from build123d import *

# Parameters (mm, degrees)
SKETCH_2_R   = 4
SKETCH_2_R_2 = 3.5


with BuildPart() as part:
    # По траектории1: sweep along a path in Эскиз1
    with BuildLine(Plane.XY) as sweep_1_path:
        Line((-12.67059026, 57.046486939), (-18.171515217, 27.990319213))
        ThreePointArc((-18.171515217, 27.990319213), (-18.041069279, 23.679327915), (-16.107188295, 19.824231748))
        Line((-16.107188295, 19.824231748), (-6.305926251, 7.761140001))
        Line((-6.305926251, 7.761140001), (0, 0))
    # Эскиз2 → По траектории1 (sweep)
    with BuildSketch(Plane(origin=(0, 0, 0), x_dir=(-0.7761140001162656, -0.6305926250944656, 0), z_dir=(0.6305926250944656, -0.7761140001162656, 0))):
        Circle(SKETCH_2_R)
        Circle(SKETCH_2_R_2, mode=Mode.SUBTRACT)
    sweep(path=sweep_1_path.line)


solid = part.part
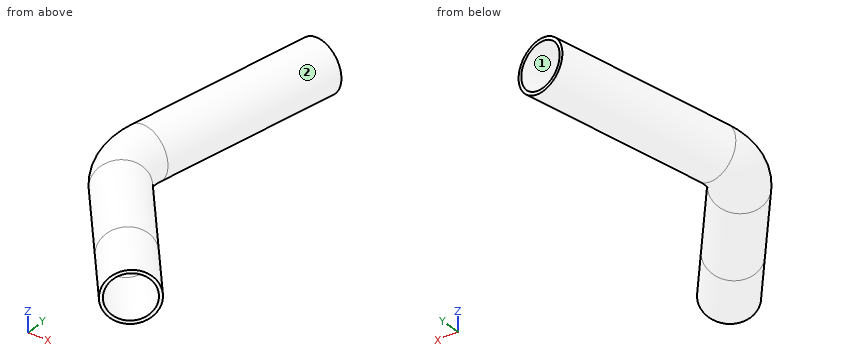
Input: part model. Units: mm. Frame: model coordinates. Face numbers are marked on the shaded views. Give positions to 0.01 mm unless a question says otherwise; leave off trailing zeros. Write each loop counter-clockwise with the first axis right and the second up, starting at its lowest first coordinate (ties: lowest second). Pieces come first, ordered by that corner, then holes. Notation, with made-up numbers: (-31, 3) -> (-26, 3) arc R23 cw to (-26, 22) -> close; hole circle Ø5 at (33.25, 69.25). An arc over 180 degrees is marked (long way). Use one line per item in the form item = value. Start each with the question number.
1) Ray query, probe 1 along Z at (x, y) = (1.75, 2); probe 2 along Z at (x, y) = (-17, 30); probe 3 along X at (y, z) = (53, 1.25). Return the intervals inside material, ascending. Write a range as from..to.
2) Section query B-B on x = -11. Count the separate pieces of the cut face and the enclosed holes in it, then the cut area to 3 significant figures.
3) Draft query along X for the marked faces 1 and 2. Return one class per face: pulls with the +X half, pulls with the -X half, needs draft (parallel to the pull), parting line crosses it, or undercut.
4) Section query C-C on z = 2. Return the cut outline in (x, y), then the cut area to 3 significant figures.
5) Section query A-A on z = -2.5. Return the cut outline in (x, y) (1 decimal), then the cut area to 3 significant figures.
6) Pin query (flat end, axial travel): pin 1 (8 mm diameter, centred on x = -11, y = 6.5, fed in from -Z); pin 2 (1.5 mm diameter, centred on x = -5, z = -0.5, fed in from +Y); pin 3 (2 mm diameter, centred on y = 13, z = -2.5, fed in from +X). Return the tip coordinate at first contact, or that it passes through.
Outcome:
q1.probe_1 = -3.02..-2.32, 2.32..3.02
q1.probe_2 = -3.92..-3.41, 3.41..3.92
q1.probe_3 = -17.3..-16.76, -10.11..-9.57
q2.separate_pieces = 2
q2.enclosed_holes = 1
q2.area = 40.9 mm^2
q3.face_1 = undercut
q3.face_2 = parting line crosses it
q4.outline = (-21.58, 28.63) arc R13.46 ccw to (-18.8, 17.64) -> (-2.69, -2.18) -> (-2.23, -1.81) -> (-18.34, 18.01) arc R12.87 cw to (-20.99, 28.52) -> (-15.49, 57.58) -> (-16.07, 57.69) -> close; (-15.35, 27.46) arc R7.13 ccw to (-13.88, 21.64) -> (2.23, 1.81) -> (2.69, 2.18) -> (-13.42, 22.01) arc R6.54 cw to (-14.77, 27.35) -> (-9.27, 56.4) -> (-9.85, 56.51) -> close
q4.area = 75.5 mm^2
q5.outline = (-21.2, 28.6) arc R13.1 ccw to (-18.5, 17.9) -> (-2.4, -2) -> (-1.9, -1.5) -> (-18, 18.3) arc R12.4 cw to (-20.6, 28.4) -> (-15.1, 57.5) -> (-15.7, 57.6) -> close; (-15.8, 27.5) arc R7.6 ccw to (-14.2, 21.4) -> (1.9, 1.5) -> (2.4, 2) -> (-13.7, 21.8) arc R6.9 cw to (-15.1, 27.4) -> (-9.6, 56.5) -> (-10.3, 56.6) -> close
q5.area = 85.9 mm^2
q6.pin_1 = -3.98
q6.pin_2 = 13.38
q6.pin_3 = -5.38
